Work out the finished part from the listing and answer in its coordinate system (mm). A direction names the side the tool comes from. Round coordinates to 2 decimals unless told otherwise and drop trailing zeros. Loops run counter-clockwise (first coordinate to the right, second up) from the corner with the lowest first, then second, coordinate; pieces in that order, holes last.
from build123d import *

# Parameters (mm, degrees)
BOSS_EXTRUDE1_REACH      = 38
BOSS_EXTRUDE1_END_RADIUS = 13
SWEEP1_PROFILE_R         = 6
CUT_SWEEP1_PROFILE_R     = 5
CUT_EXTRUDE7_REACH       = 38
CUT_EXTRUDE7_END_RADIUS  = 11
SKETCH111_R              = 1
SKETCH112_R              = 5
SKETCH112_R_2            = 1.5
BOSS_EXTRUDE2_DEPTH      = 5
BOSS_EXTRUDE3_REACH      = 24
BOSS_EXTRUDE3_END_RADIUS = 6
SKETCH113_R              = 2.5
CUT_EXTRUDE8_REACH       = 24
CUT_EXTRUDE8_END_RADIUS  = 5
SKETCH114_R              = 1


with BuildPart() as part:
    # Sketch1 → Revolve1 (revolve)
    with BuildSketch(Plane.XY):
        with BuildLine():
            Line((11, 8), (11, 24))
            Line((11, 24), (14, 24))
            Line((14, 24), (14, 21))
            ThreePointArc((14, 21), (13.292893219, 20.707106781), (13, 20))
            Line((13, 20), (13, 7))
            ThreePointArc((13, 7), (12.707106781, 6.292893219), (12, 6))
            Line((12, 6), (3, 6))
            Line((3, 6), (3, 3))
            Line((3, 3), (7, 3))
            Line((7, 3), (7, 0))
            Line((7, 0), (1, 0))
            Line((1, 0), (1, 8))
            Line((1, 8), (11, 8))
        make_face()
    revolve(axis=Axis((0, -17.809326976, 0), (0, 1, 0)))

    # Boss-Extrude1: up to this cylinder (the profile starts outside it)
    boss_extrude1_end = Plane(origin=(0, 11.178288, 0), z_dir=(0, -1, 0)) * Cylinder(BOSS_EXTRUDE1_END_RADIUS, 103, mode=Mode.PRIVATE)
    # Sketch43 → Boss-Extrude1 (add, up to the surface)
    with BuildSketch(Plane(origin=(22, 0, 0), x_dir=(0, 0, -1), z_dir=(1, 0, 0)), mode=Mode.PRIVATE) as boss_extrude1_sk1:
        with BuildLine():
            Line((-1, 16), (1, 16))
            Line((1, 16), (1, 14.872983346))
            ThreePointArc((1, 14.872983346), (0, 7), (-1, 14.872983346))
            Line((-1, 14.872983346), (-1, 16))
        make_face()
    boss_extrude1_tool1 = extrude(boss_extrude1_sk1.sketch, amount=-BOSS_EXTRUDE1_REACH, mode=Mode.PRIVATE) - boss_extrude1_end
    add(boss_extrude1_tool1.solids().sort_by_distance((22, 11.178288, 0))[0])

    # Sweep1: sweep along a path in Sketch45
    with BuildLine(Plane.XY) as sweep1_path:
        Line((25, 39), (25, 4))
        ThreePointArc((25, 4), (27.928932188, -3.071067812), (35, -6))
        Line((35, -6), (43, -6))
    # Sweep1 profile (on start of the path) → Sweep1 (sweep)
    with BuildSketch(Plane(origin=(25, 39, 0), x_dir=(0, 0, -1), z_dir=(0, -1, 0))):
        Circle(SWEEP1_PROFILE_R)
    sweep(path=sweep1_path.line)

    # Cut-Sweep1: sweep along a path in Sketch45_2
    with BuildLine(Plane.XY) as cut_sweep1_path:
        Line((25, 39), (25, 4))
        ThreePointArc((25, 4), (27.928932188, -3.071067812), (35, -6))
        Line((35, -6), (43, -6))
    # Cut-Sweep1 profile (on start of the path) → Cut-Sweep1 (sweep, cut)
    with BuildSketch(Plane(origin=(25, 39, 0), x_dir=(0, 0, -1), z_dir=(0, -1, 0))):
        Circle(CUT_SWEEP1_PROFILE_R)
    sweep(path=cut_sweep1_path.line, mode=Mode.SUBTRACT)

    # Cut-Extrude7: up to this cylinder (the profile starts outside it)
    cut_extrude7_end = Plane(origin=(0, 11, 0), z_dir=(0, -1, 0)) * Cylinder(CUT_EXTRUDE7_END_RADIUS, 99, mode=Mode.PRIVATE)
    # Sketch111 → Cut-Extrude7 (cut, up to the surface)
    with BuildSketch(Plane(origin=(22, 0, 0), x_dir=(0, 0, -1), z_dir=(1, 0, 0)), mode=Mode.PRIVATE) as cut_extrude7_sk1:
        with Locations((0, 11)):
            Circle(SKETCH111_R)
    cut_extrude7_tool1 = extrude(cut_extrude7_sk1.sketch, amount=-CUT_EXTRUDE7_REACH, mode=Mode.PRIVATE) - cut_extrude7_end
    add(cut_extrude7_tool1.solids().sort_by_distance((22, 11, 0))[0], mode=Mode.SUBTRACT)

    # Sketch112 → Boss-Extrude2 (add)
    with BuildSketch(Plane(origin=(0, 39, 0), x_dir=(1, 0, 0), z_dir=(0, 1, 0))):
        with BuildLine():
            Line((37.227272727, 2.737480895), (28.068181818, 6.843702239))
            ThreePointArc((28.068181818, 6.843702239), (25, 7.5), (21.931818182, 6.843702239))
            Line((21.931818182, 6.843702239), (12.772727273, 2.737480895))
            ThreePointArc((12.772727273, 2.737480895), (11, 0), (12.772727273, -2.737480895))
            Line((12.772727273, -2.737480895), (21.931818182, -6.843702239))
            ThreePointArc((21.931818182, -6.843702239), (25, -7.5), (28.068181818, -6.843702239))
            Line((28.068181818, -6.843702239), (37.227272727, -2.737480895))
            ThreePointArc((37.227272727, -2.737480895), (39, 0), (37.227272727, 2.737480895))
        make_face()
        with Locations(Location((25, 0, 0), (0, 0, 180))):  # turned: the seam where the file's is
            Circle(SKETCH112_R, mode=Mode.SUBTRACT)
        with Locations(Location((36, 0, 0), (0, 0, 270))):  # turned: the seam where the file's is
            Circle(SKETCH112_R_2, mode=Mode.SUBTRACT)
        with Locations(Location((14, 0, 0), (0, 0, 270))):  # turned: the seam where the file's is
            Circle(SKETCH112_R_2, mode=Mode.SUBTRACT)
    extrude(amount=BOSS_EXTRUDE2_DEPTH)

    # Boss-Extrude3: up to this cylinder (the profile starts outside it)
    boss_extrude3_end = Plane(origin=(25, 29, 0), z_dir=(0, -1, 0)) * Cylinder(BOSS_EXTRUDE3_END_RADIUS, 61, mode=Mode.PRIVATE)
    # Sketch113 → Boss-Extrude3 (add, up to the surface)
    with BuildSketch(Plane.XY.offset(8), mode=Mode.PRIVATE) as boss_extrude3_sk1:
        with Locations((25, 29)):
            Circle(SKETCH113_R)
    boss_extrude3_tool1 = extrude(boss_extrude3_sk1.sketch, amount=-BOSS_EXTRUDE3_REACH, mode=Mode.PRIVATE) - boss_extrude3_end
    add(boss_extrude3_tool1.solids().sort_by_distance((25, 29, 8))[0])

    # Cut-Extrude8: up to this cylinder (the profile starts outside it)
    cut_extrude8_end = Plane(origin=(25, 29, 0), z_dir=(0, -1, 0)) * Cylinder(CUT_EXTRUDE8_END_RADIUS, 59, mode=Mode.PRIVATE)
    # Sketch114 → Cut-Extrude8 (cut, up to the surface)
    with BuildSketch(Plane.XY.offset(8), mode=Mode.PRIVATE) as cut_extrude8_sk1:
        with Locations((25, 29)):
            Circle(SKETCH114_R)
    cut_extrude8_tool1 = extrude(cut_extrude8_sk1.sketch, amount=-CUT_EXTRUDE8_REACH, mode=Mode.PRIVATE) - cut_extrude8_end
    add(cut_extrude8_tool1.solids().sort_by_distance((25, 29, 8))[0], mode=Mode.SUBTRACT)


solid = part.part
Item 1: Section A-A, the plane x = 0 is taken. Give the vertices of the cut face in (y, z), plus the area to 3 significant figures.
Item 2: Section C-C, the plane x = 18 is taken. Give the vertices of the cut face in (y, z), plus the area to 3 significant figures.
Item 3: Straight lines are drawn through the part: line 1 (X direction, y = 18.5, z = 0); line 2 (X direction, y = 40.35, z = 0); line 3 (Y direction, x = -3.5, z = -5.5). For each, find the intervals that lie inside material, in ascending order.
Item 4: Determine the mould class of faces 1 (the face through (39, 41, 0)), 2 (the face through (-0.1, 0, 1.5)), 3 (the face through (-3, 4, 0)), 4 (the face through (0, 8, 2)) for opening direction Y: pulls with the +Y half, pulls with the -Y half, needs draft (parallel to the pull), parting line crosses it, or undercut.
Item 5: For faces 5 (the face through (10.492, 16.112, -3.304)), 6 (the face through (17.42, 41.46, -4.82)), 7 (the face through (16, 10, 0)), 8 (the face through (39.056, -11.857, 1.301)), 9 (the face through (17.288, 41.465, 4.762)), determine the directions among +Z, -Z, +X, -X, +Y, -Y from which every point of the face is accessible in a straight line to the end or side of a thin tool.
Item 6: Section D-D, the plane y = 23 is taken. Give the vertices of the cut face in (x, z).
Item 7: Section B-B, the plane y = 11 is taken. Give the vertices of the cut face in (x, z), plus the area to 3 significant figures.
Item 8: Each of these flat-tipped pins is pushed along its axis until it touches: P1, Ø6, axis at x = -7, y = 11.5, coming from the -Z side; P2, Ø0.9, axis at x = 16, y = 15.5, coming from the -Z side; P3, Ø10, axis at x = 9.5, y = 20.5, coming from the -Z side. Where does it stop, or does it pass through?
Answer below:
1. outline: (0, -7) - (3, -7) - (3, -3) - (6, -3) - (6, -12) arc R1 ccw to (7, -13) - (20, -13) arc R1 cw to (21, -14) - (24, -14) - (24, -11) - (8, -11) - (8, -1) - (0, -1) - close; (0, 1) - (8, 1) - (8, 11) - (24, 11) - (24, 14) - (21, 14) arc R1 cw to (20, 13) - (7, 13) arc R1 ccw to (6, 12) - (6, 3) - (3, 3) - (3, 7) - (0, 7) - close
1. area: 166 mm2
2. outline: (14.87, -1) - (16, -1) - (16, 1) - (14.87, 1) arc R4 ccw (long way) to start; (39, -5.08) - (44, -5.08) - (44, 5.08) - (39, 5.08) - close; hole circle Ø2 at (11, 0)
2. area: 100 mm2
3. line 1: x = -13 to -11, 11 to 13, 19 to 20, 30 to 31
3. line 2: x = 11 to 12.5, 15.5 to 20, 30 to 34.5, 37.5 to 39
3. line 3: y = 0 to 3, 6 to 8
4. face 1: needs draft
4. face 2: pulls with the -Y half
4. face 3: undercut
4. face 4: pulls with the +Y half
5. face 5: +Y
5. face 6: -Z, -X, +Y
5. face 7: none
5. face 8: +X
5. face 9: +Z, -X, +Y
6. outline: circle Ø28 at (0, 0); circle Ø12 at (25, 0); hole circle Ø22 at (0, 0); hole circle Ø10 at (25, 0)
7. outline: (12.37, -4) - (20.53, -4) arc R6 ccw (long way) to (20.53, 4) - (12.37, 4) arc R13 ccw (long way) to start; hole (10.95, -1) - (20.1, -1) arc R5 ccw (long way) to (20.1, 1) - (10.95, 1) arc R11 ccw (long way) to start
7. area: 221 mm2
8. P1: stops at z = -12.37
8. P2: stops at z = -1
8. P3: stops at z = -13.25
